```python
from build123d import *

# Parameters (mm, degrees)
PER_AGE1_D     = 5
PER_AGE1_DEPTH = 20
PER_AGE1_TIP   = 1.502151548


with BuildPart() as part:
    # Esquisse1 → Base-Révolution (revolve)
    with BuildSketch(Plane.XY, mode=Mode.PRIVATE) as base_r_volution_sk:
        Polygon((0, 0), (0, 2.5), (6, 2.5), (6, 3), (38, 3), (38, 5.875), (205, 5.875), (205, 0), align=None)
    revolve(base_r_volution_sk.sketch.rotate(Axis((0, 0, 0), (1, 0, 0)), 90), axis=Axis((0, 0, 0), (1, 0, 0)))

    # Perçage1
    with Locations(Plane(origin=(205, 0, 0), x_dir=(0, 0, -1), z_dir=(1, 0, 0))):
        with Locations((0, 0)):
            Hole(PER_AGE1_D / 2, depth=PER_AGE1_DEPTH)
            with Locations((0, 0, -(PER_AGE1_DEPTH + PER_AGE1_TIP / 2))):  # 118° drill point
                Cone(0, PER_AGE1_D / 2, PER_AGE1_TIP, mode=Mode.SUBTRACT)


solid = part.part
```
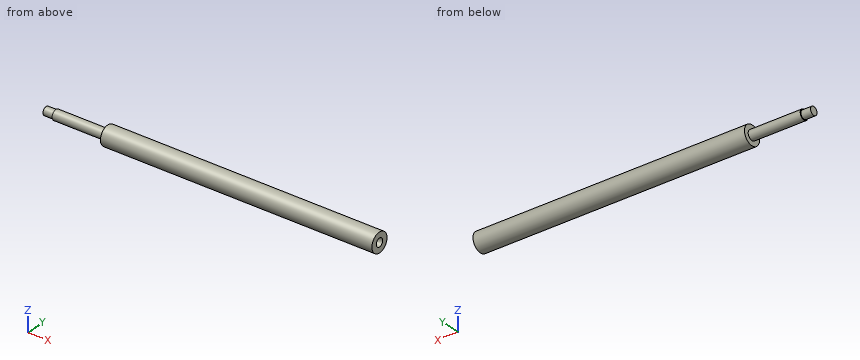
Can you work these out from the model? Positions are in its coordinate system, mm. Coordinates: 2 decimals unless noted, no trailing zeros. Loops run counter-clockwise (first coordinate to the right, second up) from the corner with the lowest first, then second, coordinate; pieces in that order, holes last.
Item 1: Please list where these lines run through material, in increasing order: L1, parallel to Y at x = 191, z = 0 (3 decimals); L2, parallel to X at y = -5, z = 2.25; L3, parallel to X at y = 1.75, z = 2.25.
Answers below:
L1: y = -5.875 to -2.5, 2.5 to 5.875
L2: x = 38 to 205
L3: x = 6 to 205
Item 2: Suppose I cut it at B-B (x = 20.5). Please give me the cut outline in (y, z), then the cut area to 3 significant figures.
Answers below:
outline: circle Ø6 at (0, 0)
area: 28.3 mm2
Item 3: Suppose I cut it at A-A (x = 83.5). Please give me the cut outline in (y, z) (3 decimals), then the cut area to 3 significant figures.
Answers below:
outline: circle Ø11.75 at (0, 0)
area: 108 mm2
Item 4: I'm going to push flat-ended pins straight in: pin 1 (5 mm diameter, centred on y = -0.5, z = 1, fed in from -X); pin 2 (6 mm diameter, centred on x = 108, y = -3.5, fed in from -Z). Where does each tip first touch, or does it pass through?
Answers below:
pin 1: stops at x = 0
pin 2: stops at z = -5.85
